Work out the finished part from the listing and answer in its coordinate system (mm). Face numbers are marked on the shaded views. A direction names the side the tool comes from. Round coordinates to 2 decimals unless told otherwise and drop trailing zeros. Order: outer loops, then holes, each group sorted by start corner. A loop starts at its lowest first (then second) coordinate and runs counter-clockwise, first axis right, second up. Notation, with made-up numbers: (50.5, 42.5) -> (106.5, 42.5) arc R24 cw to (106.5, 60.5) -> close; hole circle Ø9 at (68, 28.5). An arc over 180 degrees is marked (long way). Use a Markdown table: item, result. Add a question column.
Item 1: A cutting plane is placed at B-B, the plane z = 8. Determine the outline of the cut face in (x, y), plus the area to 3 significant figures.
Item 2: A cutting plane is placed at C-C, the plane z = -24. Determine the outline of the cut face in (x, y).
Item 3: A cutting plane is placed at A-A, the plane x = 38.5. Determine the outline of the cut face in (y, z) (3 decimals), plus the area to 3 significant figures.
Item 4: For a pull along Z with two mould halves and no side action, classify the marked faces 5, 6 and 7 as +Z half, -Z half, draft (parallel to the pull), parting line (faces both ways), or undercut.
Item 5: A tool of negligible diameter and unlimited length cuts with its end or side. For the marked faces 1, 2, 3 and 4, from which of +Z, -Z, +X, -X, +Y, -Y can it reach the whole face along a straight path? Write none if from no direction.
Item 6: Find the intervals of material crossed by L1, parallel to Y at x = 12.5, z = 9.5; L2, parallel to X at y = 1.5, z = 9; L3, parallel to Y at x = 29.5, z = -10.5, in increasing order. Write a range as [from, to].
Item 7: Flat-ended cylindrical pins translate along their axes: P1, Ø1.8, axis at x = -13, y = 13, coming from the +Z side; P2, Ø5, axis at x = -12.5, y = -12.5, coming from the -Z side; P3, Ø4, axis at y = 4.5, z = -13, coming from the -X side; P4, Ø8, axis at y = -16.5, z = -37, coming from the -X side. Find the tip coordinate at first contact, or state that the pin passes through.
Item 8: A cutting plane is placed at D-D, the plane z = -43.5. Determine the outline of the cut face in (x, y), plus the area to 3 significant figures.
from build123d import *

# Parameters (mm, degrees)
F0_W      = 95
F0_H      = 60
F1_DEPTH  = 15
F3_DEPTH  = 15
F5_W      = 13.25
F5_H      = 6.05
F6_DEPTH  = 10
F7_W      = 8
F7_H      = 8
F8_DEPTH  = 29
F11_DEPTH = 93
F12_SIZE  = 3
F14_DEPTH = 4
F15_R     = 3
F16_DEPTH = 6
F17_R     = 2
F18_R     = 4


with BuildPart() as f1:
    # F0 (on Top) → F1 (new body)
    with BuildSketch(Plane.XY):
        Rectangle(F0_W, F0_H)
    extrude(amount=F1_DEPTH)

    # F2 (on Front) → F3 (join, symmetric)
    with BuildSketch(Plane.XZ):
        with BuildLine():
            Line((-3.075, 0), (-46.235655491, 0))
            Line((-46.235655491, 0), (-46.235655491, -54))
            Line((-46.235655491, -54), (-33.9247505976, -54))
            Line((-33.9247505976, -54), (-32, -32))
            ThreePointArc((-32, -32), (-23.6896601917, -10.4872131048), (-3.075, -0.1480867922))
            Line((-3.075, -0.1480867922), (-3.075, 0))
        make_face()
        with BuildLine():
            Line((3.075, 0), (3.075, -0.1480867922))
            ThreePointArc((3.075, -0.1480867922), (23.6896601917, -10.4872131048), (32, -32))
            Line((32, -32), (33.9247505976, -54))
            Line((33.9247505976, -54), (46.235655491, -54))
            Line((46.235655491, -54), (46.235655491, 0))
            Line((46.235655491, 0), (3.075, 0))
        make_face()
    extrude(amount=F3_DEPTH, both=True)

    # F5 (on offset) → F6 (cut, symmetric)
    with BuildSketch(Plane.YZ.offset(-32)):
        with Locations((2.875, -32)):
            Rectangle(F5_W, F5_H)
    extrude(amount=F6_DEPTH, both=True, mode=Mode.SUBTRACT)

    # F7 (on Top) → F8 (cut, symmetric)
    with BuildSketch(Plane.XY):
        with Locations((-37, 4)):
            Rectangle(F7_W, F7_H)
    extrude(amount=F8_DEPTH, both=True, mode=Mode.SUBTRACT)

    # F9: F1 across plane


with BuildPart() as f1_1:
    add(f1.part)
    add(f1.part.mirror(Plane.YZ), mode=Mode.INTERSECT)

    # F10 (on face) → F11 (cut)
    with BuildSketch(Plane.YZ.offset(46.235655491)):
        with BuildLine():
            Line((-7, -20), (-7, 0))
            Line((-7, 0), (-15, 0))
            Line((-15, 0), (-15, -46))
            ThreePointArc((-15, -46), (-8.8897891542, -33.6492956449), (-7, -20))
        make_face()
    extrude(amount=-F11_DEPTH, mode=Mode.SUBTRACT)

    # F12
    f12_edges = [f1_1.edges().sort_by_distance(p)[0] for p in [
        (40.080203, -15, -54),
        (-40.080203, -15, -54),
        (0, -30, 0),
        (0, 30, 0),
        (40.080203, 15, -54),
        (-40.080203, 15, -54),
    ]]
    chamfer(f12_edges, length=F12_SIZE)

    # F13 (on face) → F14 (cut)
    with BuildSketch(Plane.XY.offset(15)):
        with BuildLine():
            Line((-12, 30), (-12, 21.9317121995))
            ThreePointArc((-12, 21.9317121995), (-25, 0), (-12, -21.9317121995))
            Line((-12, -21.9317121995), (-12, -30))
            Line((-12, -30), (12, -30))
            Line((12, -30), (12, -21.9317121995))
            ThreePointArc((12, -21.9317121995), (25, 0), (12, 21.9317121995))
            Line((12, 21.9317121995), (12, 30))
            Line((12, 30), (-12, 30))
        make_face()
    extrude(amount=-F14_DEPTH, mode=Mode.SUBTRACT)

    # F15 (on face) → F16 (cut)
    with BuildSketch(Plane.XY.offset(11)):
        with Locations((12.5, -12.5)):
            Circle(F15_R)
        with Locations((-12.5, -12.5)):
            Circle(F15_R)
        with Locations((-12.5, 12.5)):
            Circle(F15_R)
        with Locations((12.5, 12.5)):
            Circle(F15_R)
    extrude(amount=-F16_DEPTH, mode=Mode.SUBTRACT)

    # F17
    f17_edges = [f1_1.edges().sort_by_distance(p)[0] for p in [
        (-25, 0, 11),
        (25, 0, 11),
        (-12, -25.965856, 11),
        (12, -25.965856, 11),
        (12, 25.965856, 11),
        (-12, 25.965856, 11),
    ]]
    fillet(f17_edges, radius=F17_R)

    # F18 (call 1 of 4: OpenCascade refuses the feature's edges together)
    f18_edges = [f1_1.edges().sort_by_distance(p)[0] for p in [
        (-24.655328, -7, 0),
    ]]
    fillet(f18_edges, radius=F18_R)

    # F18#2 (call 2 of 4)
    f18_2_edges = [f1_1.edges().sort_by_distance(p)[0] for p in [
        (24.655328, -7, 0),
    ]]
    fillet(f18_2_edges, radius=F18_R)

    # F18#3 (call 3 of 4)
    f18_3_edges = [f1_1.edges().sort_by_distance(p)[0] for p in [
        (24.655328, 15, 0),
    ]]
    fillet(f18_3_edges, radius=F18_R)

    # F18#4 (call 4 of 4)
    f18_4_edges = [f1_1.edges().sort_by_distance(p)[0] for p in [
        (-24.655328, 15, 0),
    ]]
    fillet(f18_4_edges, radius=F18_R)


solid = f1_1.part
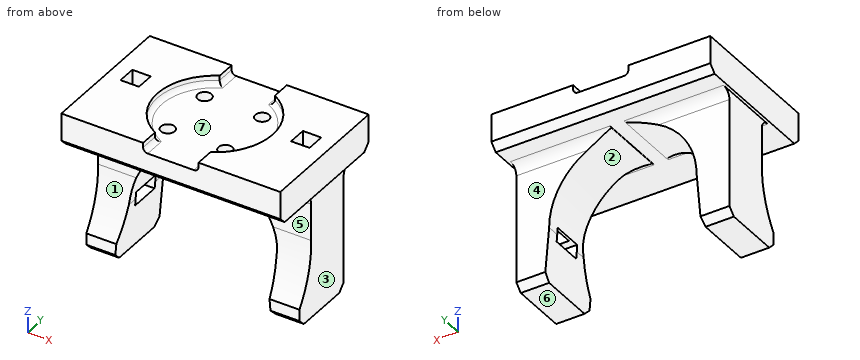
Reported:
| question | item | result |
|---|---|---|
| 1 | outline | (-47.5, -30) -> (47.5, -30) -> (47.5, 30) -> (-47.5, 30) -> close; hole (-41, 0) -> (-33, 0) -> (-33, 8) -> (-41, 8) -> close; hole circle Ø6 at (-12.5, -12.5); hole circle Ø6 at (-12.5, 12.5); hole circle Ø6 at (12.5, -12.5); hole circle Ø6 at (12.5, 12.5); hole (33, 0) -> (41, 0) -> (41, 8) -> (33, 8) -> close |
| 1 | area | 5,460 mm² |
| 2 | outline | (-46.24, -7.09) -> (-30.98, -7.09) -> (-30.98, 15) -> (-46.24, 15) -> close; (30.98, -7.09) -> (46.24, -7.09) -> (46.24, 15) -> (30.98, 15) -> close; hole (-41, 0) -> (-33, 0) -> (-33, 8) -> (-41, 8) -> close; hole (33, 0) -> (41, 0) -> (41, 8) -> (33, 8) -> close |
| 3 | outline | (-30, 3) -> (-27, 0) -> (-11, 0) arc R4 cw to (-7, -4) -> (-7, -20) arc R43 cw to (-15, -46) -> (-15, -51) -> (-12, -54) -> (12, -54) -> (15, -51) -> (15, -4) arc R4 cw to (19, 0) -> (27, 0) -> (30, 3) -> (30, 15) -> (8, 15) -> (8, -28.975) -> (9.5, -28.975) -> (9.5, -35.025) -> (-3.75, -35.025) -> (-3.75, -28.975) -> (0, -28.975) -> (0, 15) -> (-30, 15) -> close |
| 3 | area | 1,770 mm² |
| 4 | face 5 | undercut |
| 4 | face 6 | -Z half |
| 4 | face 7 | +Z half |
| 5 | face 1 | +X, -X, -Y |
| 5 | face 2 | -Z, +Y, -Y |
| 5 | face 3 | -Z, +X, +Y, -Y |
| 5 | face 4 | -Z, +X, -X, +Y |
| 6 | L1 | [-30, -15.5], [-9.5, 9.5], [15.5, 30] |
| 6 | L2 | [-47.5, -41], [-33, 33], [41, 47.5] |
| 6 | L3 | [-7, 15] |
| 7 | P1 | z = 5 |
| 7 | P2 | z = -0.13 |
| 7 | P3 | x = -46.24 |
| 7 | P4 | through |
| 8 | outline | (-46.24, -13.34) -> (-33.01, -13.34) -> (-33.01, 15) -> (-46.24, 15) -> close; (33.01, -13.34) -> (46.24, -13.34) -> (46.24, 15) -> (33.01, 15) -> close |
| 8 | area | 750 mm² |
